Read the model definition and answer for the solid it produces. Units are mm, in the model's axes. A direction names the side the tool comes from. Coordinates: 2 decimals unless noted, no trailing zeros. Order: outer loops, then holes, each group sorted by start corner. A loop starts at its lowest first (then second) coordinate and runs counter-clockwise, first axis right, second up. Notation, with made-up numbers: (66.25, -12) - (77.25, -12) arc R27 ccw to (77.25, 24) - close; hole circle Ø7 at (46.25, 5.25). An arc over 180 degrees is marked (long way). Use one line per item in the form item = value. Start each with the question number.
from build123d import *


with BuildPart() as part:
    # Sketch1 → Revolve1 (revolve)
    with BuildSketch(Plane.XY):
        with BuildLine():
            Line((-35.56, 0), (-35.56, 2.54))
            Line((-35.56, 2.54), (-30.48, 2.54))
            ThreePointArc((-30.48, 2.54), (-26.304048777, 11.979953655), (-16.51, 15.24))
            Line((-16.51, 15.24), (0, 15.24))
            Line((0, 15.24), (0, 6.427550656))
            Line((0, 6.427550656), (-2.54, 6.427550656))
            Line((-2.54, 6.427550656), (-2.54, 11.43))
            Line((-2.54, 11.43), (-22.759122002, 11.43))
            ThreePointArc((-22.759122002, 11.43), (-24.989007002, 9.723072017), (-26.67, 7.473571452))
            Line((-26.67, 7.473571452), (-26.67, 0))
            Line((-26.67, 0), (-35.56, 0))
        make_face()
    revolve(axis=Axis((0, 15.24, 0), (0, -1, 0)))


solid = part.part
Q1. A cutting plane is placed at C-C (y = 10). Give the vertices of the cut face in (x, z), then the cut area to 3 significant figures.
Q2. A cutting plane is placed at D-D (y = 4.5). Give the vertices of the cut face in (x, z), then the cut area to 3 significant figures.
Q3. Consider probe 1 along Z at (x, y) = (0, 2.5); probe 2 along X at (y, z) = (10, -18.5); probe 3 along Z at (x, y) = (-21.5, 5.5). Determine where each line is inside the solid, lowest interval first.
Q4. A cutting plane is placed at B-B (z = 0). Give the vertices of the cut face in (x, y).
Q5. Given P1, Ø3, axis at x = 2, y = 4, coming from the -Z side; P2, Ø16.5, axis at x = 0.5, z = 1.5, coming from the +Y side; P3, Ø23, axis at x = 3.5, z = 9, coming from the -Y side, each flat-ended and moving along its own axis, determine where each tip first touches the part or whether it passes through.
Q6. Which of the six approach directions +Z, -Z, +X, -X, +Y, -Y give full straight-line access (tool end or side, diameter ignored) to faces 1 (the flat face through (5, 11.43, 0)), 2 (the flat face through (-26.2, 2.54, -16))?
Q7. A cutting plane is placed at A-A (x = 0). Give the vertices of the cut face in (y, z).
Q8. For a pull along Z with two mould halves and no side action, classify faces 3 (the flat face through (5, 0, -27)), 4 (the cylindrical face through (7.709, 1.288, 34.714)), 5 (the cylindrical face through (0.33, 8.96, -2.52)) as +Z half, -Z half, draft (parallel to the pull), parting line (faces both ways), or undercut.
Result sheet:
q1.outline = circle Ø56.14 at (0, 0); circle Ø5.08 at (0, 0); hole circle Ø49.41 at (0, 0)
q1.area = 579 mm^2
q2.outline = circle Ø60.66 at (0, 0); hole circle Ø53.34 at (0, 0)
q2.area = 655 mm^2
q3.probe_1 = -35.56 to -26.67, 26.67 to 35.56
q3.probe_2 = -21.11 to -16.37, 16.37 to 21.11
q3.probe_3 = -21.11 to -15.78, 15.78 to 21.11
q4.outline = (-35.56, 0) - (-26.67, 0) - (-26.67, 7.47) arc R10.22 cw to (-22.76, 11.43) - (-2.54, 11.43) - (-2.54, 6.43) - (2.54, 6.43) - (2.54, 11.43) - (22.76, 11.43) arc R10.22 cw to (26.67, 7.47) - (26.67, 0) - (35.56, 0) - (35.56, 2.54) - (30.48, 2.54) arc R12.76 ccw to (16.51, 15.24) - (-16.51, 15.24) arc R12.76 ccw to (-30.48, 2.54) - (-35.56, 2.54) - close
q5.P1 = -35.52
q5.P2 = 15.24
q5.P3 = 6.43
q6.face_1 = -Y
q6.face_2 = +Y
q7.outline = (0, -35.56) - (2.54, -35.56) - (2.54, -30.48) arc R12.76 ccw to (15.24, -16.51) - (15.24, 16.51) arc R12.76 ccw to (2.54, 30.48) - (2.54, 35.56) - (0, 35.56) - (0, 26.67) - (7.47, 26.67) arc R10.22 cw to (11.43, 22.76) - (11.43, 2.54) - (6.43, 2.54) - (6.43, -2.54) - (11.43, -2.54) - (11.43, -22.76) arc R10.22 cw to (7.47, -26.67) - (0, -26.67) - close
q8.face_3 = draft
q8.face_4 = parting line
q8.face_5 = undercut
